Design review of the part built by this model. Coordinates are the model's own, in mm. A direction names the side the tool comes from. Round coordinates to 2 decimals unless told otherwise and drop trailing zeros. Loops run counter-clockwise (first coordinate to the right, second up) from the corner with the lowest first, then second, coordinate; pieces in that order, holes last. Notation, with made-up numbers: (-32, 71) - (-13, 71) arc R29 ccw to (-13, 98) - close; hole circle Ø10 at (47, 48.25). An arc over 180 degrees is marked (long way). Return JSON: item names as keys, results as strings. Group by question number.
(1) We need section A-A, the plane z = -6.5. Write out the cut boundary in (x, y), and give its area (3 significant figures).
(2) We need section D-D, the plane y = -2.3. Give the number of separate pieces and of enclosed holes in the cut face, and give its area (3 significant figures).
(3) Wall thickness on L1, parallel to X at y = -2.4, z = -1; L2, parallel to X at y = -1.7, z = 7; L3, parallel to X at y = -3, z = -4.5: over which ranges is each line inside the solid? List them lowest first. Write a range as [from, to].
(4) Clearance check with flat-ended pins moving along their axes: pin 1 (1.4 mm diameter, centred on x = 9.5, y = -2, fed in from -Z); pin 2 (1.4 mm diameter, centred on x = 10.5, y = -2, fed in from +Z); pin 3 (2 mm diameter, centred on x = 0, z = -3.5, fed in from +Y); pin 4 (1.7 mm diameter, centred on x = 10.5, y = -2, fed in from -Z). State where each tip first meets the part, or that it passes through.
(5) We need section B-B, the plane x = 0.5. Write out the cut boundary in (y, z).
(6) We need section C-C, the plane z = -1. Write out the cut boundary in (x, y), and give its area (3 significant figures).
(7) The part is to be moulded in two halves that separate along X. For faces 1 (the flat face through (9, -2, 5.5)), 2 (the flat face through (-10, -2, 0)), 3 (the flat face through (-11.5, -1.9, 15)), 4 (the flat face through (3, -3.81, 0)), say which applies: pulls with the +X half, pulls with the -X half, needs draft (parallel to the pull), parting line crosses it, or undercut.
(8) For faces 5 (the flat face through (9, -2, -0.2)), 6 (the flat face through (9.75, -2, 7)), 7 (the flat face through (6, -2, -14)), list the 3-axis set-ups (+Z, -Z, +X, -X, +Y, -Y) from which the entire face can be reached by the end or side of a thin tool; tool diameter is ignored.
from build123d import *

# Parameters (mm, degrees)
F1_DEPTH = 3.81


# Not quite as in the source:
# - ends of sketch curves that miss each other by under 0.0002 mm in the source are joined


with BuildPart() as f1:
    # F0 (on Front) → F1 (new body)
    with BuildSketch(Plane.XZ):
        with BuildLine():
            Line((-10.292893, -16), (-4.25, -16))
            Line((-4.25, -16), (-4.25, -14.8))
            ThreePointArc((-4.25, -14.8), (-4.9571067812, -14.5071067812), (-5.25, -13.8))
            ThreePointArc((-5.25, -13.8), (-4.9571067812, -13.0928932188), (-4.25, -12.8))
            Line((-4.25, -12.8), (-4.25, -11.8))
            Line((-4.25, -11.8), (-10, -11.8))
            Line((-10, -11.8), (-10, 11.8))
            Line((-10, 11.8), (-4.25, 11.8))
            Line((-4.25, 11.8), (-4.25, 12.8))
            ThreePointArc((-4.25, 12.8), (-4.9571067812, 13.0928932188), (-5.25, 13.8))
            ThreePointArc((-5.25, 13.8), (-4.9571067812, 14.5071067812), (-4.25, 14.8))
            Line((-4.25, 14.8), (-4.25, 16))
            Line((-4.25, 16), (-10.292893, 16))
            ThreePointArc((-10.292893, 16), (-10.4842347162, 15.9619397663), (-10.6464463906, 15.8535533906))
            Line((-10.6464463906, 15.8535533906), (-12.353554, 14.146447))
            ThreePointArc((-12.353554, 14.146447), (-12.4619399016, 13.9842353895), (-12.5, 13.792894))
            Line((-12.5, 13.792894), (-12.5, -13.792893))
            ThreePointArc((-12.5, -13.792893), (-12.4619399016, -13.9842343895), (-12.3535538906, -14.1464458906))
            Line((-12.3535538906, -14.1464458906), (-10.646447, -15.853553))
            ThreePointArc((-10.646447, -15.853553), (-10.4842350428, -15.961939631), (-10.292893, -16))
        make_face()
        with BuildLine():
            Line((12.5, -11.1), (12.5, 9))
            ThreePointArc((12.5, 9), (12.3535533906, 9.3535533906), (12, 9.5))
            Line((12, 9.5), (10.25, 9.5))
            ThreePointArc((10.25, 9.5), (9.8964466094, 9.3535533906), (9.75, 9))
            Line((9.75, 9), (9.75, 5.5))
            Line((9.75, 5.5), (8.5, 5.5))
            Line((8.5, 5.5), (8.5, 2.2))
            Line((8.5, 2.2), (9.75, 2.2))
            Line((9.75, 2.2), (9.75, -0.2))
            Line((9.75, -0.2), (8.5, -0.2))
            Line((8.5, -0.2), (8.5, -3.5))
            Line((8.5, -3.5), (5.5, -3.5))
            Line((5.5, -3.5), (5.5, -0.2))
            Line((5.5, -0.2), (4.25, -0.2))
            Line((4.25, -0.2), (4.25, 2.2))
            Line((4.25, 2.2), (5.5, 2.2))
            Line((5.5, 2.2), (5.5, 5.5))
            Line((5.5, 5.5), (4.25, 5.5))
            Line((4.25, 5.5), (4.25, 13.792894))
            ThreePointArc((4.25, 13.792894), (4.2119397663, 13.9842357162), (4.1035533906, 14.1464473906))
            Line((4.1035533906, 14.1464473906), (2.396446, 15.853554))
            ThreePointArc((2.396446, 15.853554), (2.2342343895, 15.9619399016), (2.042893, 16))
            Line((2.042893, 16), (-4.25, 16))
            Line((-4.25, 16), (-4.25, 14.8))
            ThreePointArc((-4.25, 14.8), (-3.5428932188, 14.5071067812), (-3.25, 13.8))
            ThreePointArc((-3.25, 13.8), (-3.5428932188, 13.0928932188), (-4.25, 12.8))
            Line((-4.25, 12.8), (-4.25, 11.8))
            Line((-4.25, 11.8), (1.5, 11.8))
            Line((1.5, 11.8), (1.5, -11.8))
            Line((1.5, -11.8), (-4.25, -11.8))
            Line((-4.25, -11.8), (-4.25, -12.8))
            ThreePointArc((-4.25, -12.8), (-3.5428932188, -13.0928932188), (-3.25, -13.8))
            ThreePointArc((-3.25, -13.8), (-3.5428932188, -14.5071067812), (-4.25, -14.8))
            Line((-4.25, -14.8), (-4.25, -16))
            Line((-4.25, -16), (3.792893, -16))
            ThreePointArc((3.792893, -16), (3.9842347162, -15.9619397663), (4.1464463906, -15.8535533906))
            Line((4.1464463906, -15.8535533906), (8.753553, -11.246446))
            ThreePointArc((8.753553, -11.246446), (8.9157652838, -11.1380602337), (9.107107, -11.1))
            Line((9.107107, -11.1), (12.5, -11.1))
        make_face()
    extrude(amount=F1_DEPTH)


solid = f1.part
Solutions:
{
 "1": {"outline": "(-12.5, -3.81) - (-10, -3.81) - (-10, 0) - (-12.5, 0) - close; (1.5, -3.81) - (12.5, -3.81) - (12.5, 0) - (1.5, 0) - close", "area": "51.4 mm^2"},
 "2": {"separate pieces": "1", "enclosed holes": "3", "area": "378 mm^2"},
 "3": {"L1": "[-12.5, -10], [1.5, 5.5], [8.5, 12.5]", "L2": "[-12.5, -10], [1.5, 4.25], [9.75, 12.5]", "L3": "[-12.5, -10], [1.5, 12.5]"},
 "4": {"pin 1": "z = -11.21", "pin 2": "z = 9.5", "pin 3": "through", "pin 4": "z = -11.1"},
 "5": {"outline": "(-3.81, -16) - (0, -16) - (0, -11.8) - (-3.81, -11.8) - close; (-3.81, 11.8) - (0, 11.8) - (0, 16) - (-3.81, 16) - close"},
 "6": {"outline": "(-12.5, -3.81) - (-10, -3.81) - (-10, 0) - (-12.5, 0) - close; (1.5, -3.81) - (5.5, -3.81) - (5.5, 0) - (1.5, 0) - close; (8.5, -3.81) - (12.5, -3.81) - (12.5, 0) - (8.5, 0) - close", "area": "40.0 mm^2"},
 "7": {"face 1": "undercut", "face 2": "undercut", "face 3": "pulls with the -X half", "face 4": "needs draft"},
 "8": {"face 5": "+Y, -Y", "face 6": "+Z, +Y, -Y", "face 7": "-Z, +X, +Y, -Y"}
}
